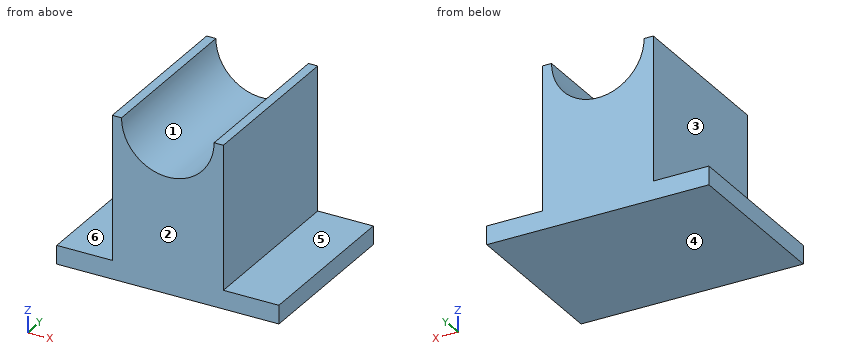
```python
from build123d import *

# Parameters (mm, degrees)
F0_W     = 152.4
F0_H     = 111.125
F1_DEPTH = 114.3
F2_W     = 38.1
F2_H     = 98.425
F3_DEPTH = 114.3
F5_DEPTH = 114.3


with BuildPart() as f1:
    # F0 (on Front) → F1 (new body)
    with BuildSketch(Plane.XZ):
        with Locations((76.2, 55.5625)):
            Rectangle(F0_W, F0_H)
    extrude(amount=F1_DEPTH)

    # F2 (on face) → F3 (cut)
    with BuildSketch(Plane.XZ.offset(114.3)):
        with Locations((19.05, 61.9125)):
            Rectangle(F2_W, F2_H)
        with Locations((133.35, 61.9125)):
            Rectangle(F2_W, F2_H)
    extrude(amount=-F3_DEPTH, mode=Mode.SUBTRACT)

    # F4 (on face) → F5 (cut)
    with BuildSketch(Plane.XZ.offset(114.3)):
        with BuildLine():
            Line((107.95, 111.125), (44.45, 111.125))
            ThreePointArc((44.45, 111.125), (76.2, 79.32702), (107.95, 111.125))
        make_face()
    extrude(amount=-F5_DEPTH, mode=Mode.SUBTRACT)


solid = f1.part
```
Read the model definition and answer for the solid it produces. Units are mm, in the model's axes. Face numbers are marked on the shaded views. A direction names the side the tool comes from. Give positions to 0.01 mm unless a question says otherwise; leave off trailing zeros. Order: outer loops, then holes, each group sorted by start corner. A loop starts at its lowest first (then second) coordinate and runs counter-clockwise, first axis right, second up.
(1) Find section C-C (x = 76.2). Give the vertices of the cut face in (y, z), plus the area to 3 significant figures.
(2) Straight lines are drawn through the part: L1, parallel to Z at x = 135.5, y = -86.5; L2, parallel to X at y = -102, z = 67.5; L3, parallel to X at y = -32, z = 98.5. For each, find the intervals that lie inside material, in ascending order.
(3) For the marked faces 4, 5 and 6, determine the directions among +Z, -Z, +X, -X, +Y, -Y from which every point of the face is accessible in a straight line to the end or side of a thin tool.
(4) For a pull along X with two mould halves and no side action, classify the marked faces 1, 2 and 3 as released by +X, released by -X, zero draft, split by the parting line, or undercut.
(5) Find section B-B (z = 97.5). Give the vertices of the cut face in (x, y), plus the area to 3 significant figures.
(6) Find section A-A (y = -103.5). Give the vertices of the cut face in (x, z) (3 decimals), plus the area to 3 significant figures.
(7) Find section D-D (z = 62). Give the vertices of the cut face in (x, y), plus the area to 3 significant figures.
(8) Given pin 1 (1.5 mm diameter, centred on y = -93.5, z = 53.5, fed in from -X); pin 2 (11.5 mm diameter, centred on x = 13, y = -59.5, fed in from +Z), each flat-ended and moving along its own axis, determine where each tip first touches the part or whether it passes through.
Result sheet:
1. outline: (-114.3, 0) - (0, 0) - (0, 79.33) - (-114.3, 79.33) - close
1. area: 9,070 mm2
2. L1: z = 0 to 12.7
2. L2: x = 38.1 to 114.3
2. L3: x = 38.1 to 47.05, 105.35 to 114.3
3. face 4: -Z, +X, -X, +Y, -Y
3. face 5: +Z, +X, +Y, -Y
3. face 6: +Z, -X, +Y, -Y
4. face 1: undercut
4. face 2: zero draft
4. face 3: released by -X
5. outline: (38.1, -114.3) - (47.5, -114.3) - (47.5, 0) - (38.1, 0) - close; (104.9, -114.3) - (114.3, -114.3) - (114.3, 0) - (104.9, 0) - close
5. area: 2,150 mm2
6. outline: (0, 0) - (152.4, 0) - (152.4, 12.7) - (114.3, 12.7) - (114.3, 111.125) - (107.95, 111.125) arc R31.75 cw to (44.45, 111.125) - (38.1, 111.125) - (38.1, 12.7) - (0, 12.7) - close
6. area: 7,850 mm2
7. outline: (38.1, -114.3) - (114.3, -114.3) - (114.3, 0) - (38.1, 0) - close
7. area: 8,710 mm2
8. pin 1: stops at x = 38.1
8. pin 2: stops at z = 12.7
